from build123d import *

# Parameters (mm, degrees)
SKETCH_2_W          = 4.549870692
SKETCH_2_H          = 5
CUT_EXTRUDE_1_DEPTH = 12
FILLET_1_R          = 2.5
FILLET_2_R          = 2.5


with BuildPart() as part:
    # 草图1 → 旋转1 (revolve)
    with BuildSketch(Plane.XY, mode=Mode.PRIVATE) as revolve_1_sk:
        Polygon((0, 0), (0, 6), (12, 6), (12, 5), (13, 5), (13, 7), (30, 7), (30, 8), (44, 8), (44, 10), (84, 10), (84, 9), (85, 9), (85, 14), (89, 14), (89, 0), align=None)
    revolve(revolve_1_sk.sketch.rotate(Axis((0, 0, 0), (-1, 0, 0)), 90), axis=Axis((0, 0, 0), (-1, 0, 0)))

    # 草图2 → 切除-拉伸1 (cut)
    with BuildSketch(Plane.ZY.offset(-28)):
        with Locations((-5.274935346, 0)):
            Rectangle(SKETCH_2_W, SKETCH_2_H)
    extrude(amount=CUT_EXTRUDE_1_DEPTH, mode=Mode.SUBTRACT)

    # 圆角1
    fillet_1_edges = [part.edges().sort_by_distance(p)[0] for p in [
        (16, -2.5, -4.769174208),
        (16, 2.5, -4.769174208),
    ]]
    fillet(fillet_1_edges, radius=FILLET_1_R - 0.0001)  # a hair under: the kernel refuses the full size

    # 圆角2
    fillet_2_edges = [part.edges().sort_by_distance(p)[0] for p in [
        (28, 2.5, -4.769174208),
        (28, -2.5, -4.769174208),
    ]]
    fillet(fillet_2_edges, radius=FILLET_2_R - 0.0001)  # a hair under: the kernel refuses the full size


solid = part.part
Input: part model. Units: mm. Frame: model coordinates. A direction names the side the tool comes from. Coordinates: 2 decimals unless noted, no trailing zeros. Loops run counter-clockwise (first coordinate to the right, second up) from the corner with the lowest first, then second, coordinate; pieces in that order, holes last.
(1) First-contact query: pin 1 Ø6 at (x, y) = (37, 9.5) entering from -Z; pin 2 Ø10 at (x, y) = (51, 7) entering from +Z; pin 3 Ø3 at (x, z) = (20.5, -4.5) entering from -Y; pin 4 Ø3 at (x, y) = (32, -11) entering from -Z. Flat tips, straight axial feed; report the tip coordinate or a pass-through.
(2) Section C-C on x = 33.5. Return the cut outline in (y, z).
(3) Material intervals for probe 1 along X at (y, z) = (2, 4.75); probe 2 along X at (y, z) = (-1.75, 9); probe 3 along Z at (x, y) = (47.5, 6), sorted ascending.
(4) Pull-direction query (X, two-part tool) for faces 5 (the face through (17, 2, -5)), 6 (the face through (0, 0, 0)), 7 (the face through (84.507, -6.083, 6.633)), 8 (the face through (37.1, 7.81, 1.73)); classes: released by +X, released by -X, zero draft, split by the parting line, or undercut.
(5) Section D-D on x = 73. Return the cut outline in (y, z), then the cut area to 3 significant figures.
(6) Set-up query: faces 1 (the face through (27, -2, -5)), 2 (the face through (13, -5, -2)), 3 (the face through (21.619, 4.259, 5.555)), 4 (the face through (87, 12.4, -6.5)). Return all of +Z, -Z, +X, -X, +Y, -Y with unobstructed straight access to the full face (end or side cutting, diameter ignored); none if empty.
(7) Section A-A on z = -1.75. Return the cut outline in (x, y), then the cut area to 3 significant figures.
Data:
1. pin 1: stops at z = -4.66
1. pin 2: stops at z = 9.8
1. pin 3: stops at y = -6.32
1. pin 4: passes through
2. outline: circle Ø16 at (0, 0)
3. probe 1: x = 0 to 12, 13 to 89
3. probe 2: x = 44 to 84, 85 to 89
3. probe 3: z = -8 to 8
4. face 5: undercut
4. face 6: released by -X
4. face 7: undercut
4. face 8: zero draft
5. outline: circle Ø20 at (0, 0)
5. area: 314 mm2
6. face 1: -Z
6. face 2: none
6. face 3: -X
6. face 4: +X, -X
7. outline: (0, -5.74) - (12, -5.74) - (12, -4.68) - (13, -4.68) - (13, -6.78) - (30, -6.78) - (30, -7.81) - (44, -7.81) - (44, -9.85) - (84, -9.85) - (84, -8.83) - (85, -8.83) - (85, -13.89) - (89, -13.89) - (89, 13.89) - (85, 13.89) - (85, 8.83) - (84, 8.83) - (84, 9.85) - (44, 9.85) - (44, 7.81) - (30, 7.81) - (30, 6.78) - (13, 6.78) - (13, 4.68) - (12, 4.68) - (12, 5.74) - (0, 5.74) - close
7. area: 1,510 mm2
